```python
from build123d import *

# Parameters (mm, degrees)
SKETCH1_W                                       = 70
SKETCH1_H                                       = 55
BOSS_EXTRUDE1_DEPTH                             = 6.35
CUT_EXTRUDE1_START                              = 6.35
SKETCH1_3_R                                     = 1
CUT_EXTRUDE1_DEPTH                              = 6.35
CSK_FOR_M3_FLAT_HEAD_MACHINE_SCREW1_D           = 3.4
CSK_FOR_M3_FLAT_HEAD_MACHINE_SCREW1_CSINK_D     = 7.3
CSK_FOR_M3_FLAT_HEAD_MACHINE_SCREW1_CSINK_ANGLE = 90
FILLET1_R                                       = 5
CSK_FOR_M5_FLAT_HEAD_MACHINE_SCREW2_D           = 5.5
CSK_FOR_M5_FLAT_HEAD_MACHINE_SCREW2_CSINK_D     = 11.4
CSK_FOR_M5_FLAT_HEAD_MACHINE_SCREW2_CSINK_ANGLE = 90


with BuildPart() as part:
    # Sketch1 → Boss-Extrude1 (new body)
    with BuildSketch(Plane(origin=(0, 0, 0), x_dir=(1, 0, 0), z_dir=(0, 1, 0))):
        with Locations((2.711596357, 0)):
            Rectangle(SKETCH1_W, SKETCH1_H)
    extrude(amount=BOSS_EXTRUDE1_DEPTH)

    # Sketch1<3> → Cut-Extrude1 (cut)
    with BuildSketch(Plane(origin=(0, 0, 0), x_dir=(1, 0, 0), z_dir=(0, 1, 0)).offset(CUT_EXTRUDE1_START)):
        with Locations(Location((30.211596357, -10, 0), (0, 0, 90))):
            Circle(SKETCH1_3_R)
        with Locations(Location((10.211596357, -10, 0), (0, 0, 90))):
            Circle(SKETCH1_3_R)
        with Locations(Location((30.211596357, 10, 0), (0, 0, 90))):
            Circle(SKETCH1_3_R)
        with Locations(Location((10.211596357, 10, 0), (0, 0, 90))):
            Circle(SKETCH1_3_R)
        with Locations(Location((1.211596357, -15.25, 0), (0, 0, 90))):
            Circle(SKETCH1_3_R)
        with Locations(Location((-24.788403643, -15.25, 0), (0, 0, 90))):
            Circle(SKETCH1_3_R)
        with Locations(Location((1.211596357, 15.25, 0), (0, 0, 90))):
            Circle(SKETCH1_3_R)
        with Locations(Location((-24.788403643, 15.25, 0), (0, 0, 90))):
            Circle(SKETCH1_3_R)
    extrude(amount=-CUT_EXTRUDE1_DEPTH, mode=Mode.SUBTRACT)

    # CSK for M3 Flat Head Machine Screw1 (through all)
    with Locations(Plane(origin=(0, 6.35, 0), x_dir=(1, 0, 0), z_dir=(0, 1, 0))):
        with Locations((30.211596357, -10), (10.211596357, -10), (10.211596357, 10), (30.211596357, 10)):
            CounterSinkHole(CSK_FOR_M3_FLAT_HEAD_MACHINE_SCREW1_D / 2, CSK_FOR_M3_FLAT_HEAD_MACHINE_SCREW1_CSINK_D / 2, counter_sink_angle=CSK_FOR_M3_FLAT_HEAD_MACHINE_SCREW1_CSINK_ANGLE)

    # Fillet1
    fillet1_edges = [part.edges().sort_by_distance(p)[0] for p in [
        (37.711596357, 3.175, 27.5),
        (37.711596357, 3.175, -27.5),
        (-32.288403643, 3.175, -27.5),
        (-32.288403643, 3.175, 27.5),
    ]]
    fillet(fillet1_edges, radius=FILLET1_R)

    # CSK for M5 Flat Head Machine Screw2 (through all)
    with Locations(Plane(origin=(0, 0, 0), x_dir=(-1, 0, 0), z_dir=(0, -1, 0))):
        with Locations((24.788403643, -15.25), (24.788403643, 15.25), (-1.211596357, 15.25), (-1.211596357, -15.25)):
            CounterSinkHole(CSK_FOR_M5_FLAT_HEAD_MACHINE_SCREW2_D / 2, CSK_FOR_M5_FLAT_HEAD_MACHINE_SCREW2_CSINK_D / 2, counter_sink_angle=CSK_FOR_M5_FLAT_HEAD_MACHINE_SCREW2_CSINK_ANGLE)


solid = part.part
```
Geometry check sheet. Reference: the model listing, model coordinates, mm. Coordinates: 2 decimals unless noted, no trailing zeros. Write each loop counter-clockwise with the first axis right and the second up, starting at its lowest first coordinate (ties: lowest second). Pieces come first, ordered by that corner, then holes. Notation, with made-up numbers: M -39.5,2.5 L -21.5,2.5 A26 cw -21.5,41.5 Z; hole C 0.5,81 d4. An arc over 180 degrees is marked long. Use one line per item in the form item = value. Start each with the question number.
1) Section check B-B on y = 1. State how many separate pieces and enclosed holes the cut face has, and give its area (3 significant figures).
2) Go/stop test with a flat-tipped pin: pin 1 Ø3.5 at (x, z) = (-24.79, 15.25) entering from +Y. Record where the tip stops, or that it passes through.
3) Section check A-A on z = 15.25. Enter the section's corners in (x, y).
4) Thickness scan on probe 1 along Z at (x, y) = (-24.5, 4.25); probe 2 along X at (y, z) = (3.5, 11); probe 3 along Z at (x, y) = (2.5, 5.25). Record the ranges inside material, lowest first. Write a range as from..to.
Responses:
q1.separate_pieces = 1
q1.enclosed_holes = 8
q1.area = 3,510 mm2
q2.pin_1 = through
q3.outline = M -32.29,0 L -30.49,0 L -27.54,2.95 L -27.54,6.35 L -32.29,6.35 Z; M -22.04,2.95 L -19.09,0 L -4.49,0 L -1.54,2.95 L -1.54,6.35 L -22.04,6.35 Z; M 3.96,2.95 L 6.91,0 L 37.71,0 L 37.71,6.35 L 3.96,6.35 Z
q4.probe_1 = -27.5..-17.98, -12.52..12.52, 17.98..27.5
q4.probe_2 = -32.29..8.84, 11.59..28.84, 31.59..37.71
q4.probe_3 = -27.5..-17.68, -12.82..12.82, 17.68..27.5
